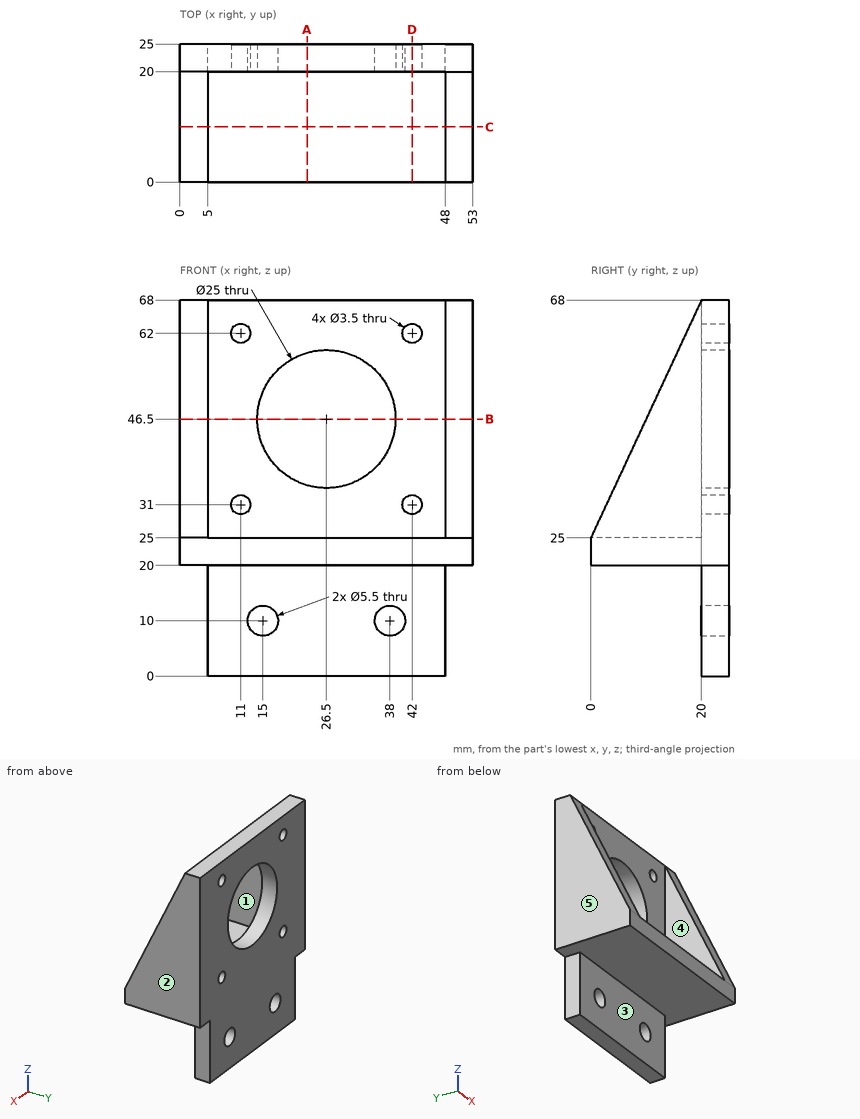
Geometry check sheet. Reference: drawing and pictorial views, mm from the part's lowest x, y, z. A direction names the side the tool comes from. Round coordinates to 2 decimals unless told otherwise and drop trailing zeros. Loops run counter-clockwise (first coordinate to the right, second up) from the corner with the lowest first, then second, coordinate; pieces in that order, holes last. Notation, with made-up numbers: (-13.5, 21) - (-9.5, 21) arc R27 cw to (-9.5, 44) - close; hole circle Ø3 at (-36.5, 68.5). An arc over 180 degrees is marked (long way). Answer in a Markdown table with one row per item. Add a question column.
Q1. Section check A-A on x = 23. Enter the section's corners in (y, z), plus the area to 3 significant figures.
Q2. Section check D-D on x = 42. Enter the section's corners in (y, z).
Q3. Material ranges on line 1 (X direction, y = 23.6, z = 62); line 2 (X direction, y = 23.1, z = 10); line 3 (X direction, y = 7.5, z = 27), recorded low to high.
Q4. Tool access check on the marked faces 4 and 5. Record the directions out of +Z, -Z, +X, -X, +Y, -Y that give a thin tool (end or side, any length) a straight path to the whole face; none if there is none.
Q5. Section check C-C on y = 10. Enter the section's corners in (x, z), plus the area to 3 significant figures.
Q6. Release check for a two-part mould opening along X. For the marked faces 1, 2 and 3 record: pulls with the +X half, pulls with the -X half, needs draft (parallel to the pull), parting line crosses it, or undercut.
Q7. Section check B-B on z = 46.5. Enter the section's corners in (x, y), plus the area to 3 significant figures.
Q8. Gauge pin test, flat ends, axial feed: pin 1 (5 mm diameter, centred on x = 45, z = 7, fed in from -Y); pin 2 (2 mm diameter, centred on y = 17.5, z = 19.5, fed in from -X); pin 3 (1.5 mm diameter, centred on x = 8.5, y = 10, fed in from -Z); pin 4 (2.5 mm diameter, centred on y = 21.5, z = 8.5, fed in from -X). Record the tip position at first contact, or that the pin passes through.
Found:
| question | item | result |
|---|---|---|
| 1 | outline | (0, 20) - (20, 20) - (20, 0) - (25, 0) - (25, 34.5) - (20, 34.5) - (20, 25) - (0, 25) - close; (20, 58.5) - (25, 58.5) - (25, 68) - (20, 68) - close |
| 1 | area | 320 mm² |
| 2 | outline | (0, 20) - (20, 20) - (20, 0) - (25, 0) - (25, 29.25) - (20, 29.25) - (20, 25) - (0, 25) - close; (20, 32.75) - (25, 32.75) - (25, 60.25) - (20, 60.25) - close; (20, 63.75) - (25, 63.75) - (25, 68) - (20, 68) - close |
| 3 | line 1 | x = 0 to 9.25, 12.75 to 40.25, 43.75 to 53 |
| 3 | line 2 | x = 5 to 12.25, 17.75 to 35.25, 40.75 to 48 |
| 3 | line 3 | x = 0 to 5, 48 to 53 |
| 4 | face 4 | +Z, -Y |
| 4 | face 5 | +Z, -Z, -X, +Y, -Y |
| 5 | outline | (0, 20) - (53, 20) - (53, 46.5) - (48, 46.5) - (48, 25) - (5, 25) - (5, 46.5) - (0, 46.5) - close |
| 5 | area | 480 mm² |
| 6 | face 1 | undercut |
| 6 | face 2 | pulls with the +X half |
| 6 | face 3 | needs draft |
| 7 | outline | (0, 10) - (5, 10) - (5, 20) - (14, 20) - (14, 25) - (0, 25) - close; (39, 20) - (48, 20) - (48, 10) - (53, 10) - (53, 25) - (39, 25) - close |
| 7 | area | 240 mm² |
| 8 | pin 1 | stops at y = 20 |
| 8 | pin 2 | stops at x = 0 |
| 8 | pin 3 | stops at z = 20 |
| 8 | pin 4 | stops at x = 5 |
